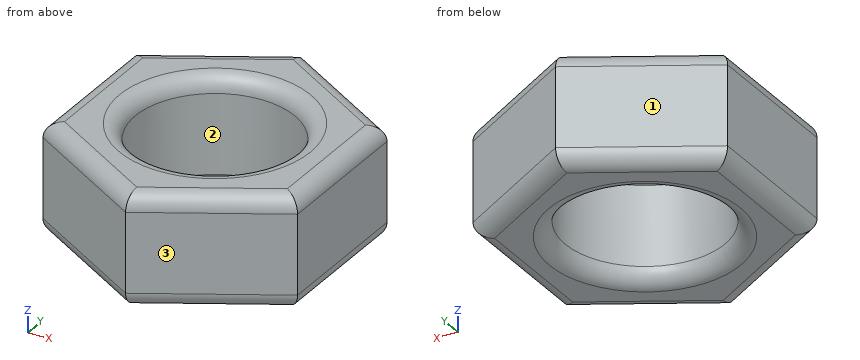
from build123d import *

# Parameters (mm, degrees)
F0_R     = 2.5
F1_DEPTH = 3.5
F2_R     = 0.5
F3_R     = 0.5


with BuildPart() as f1:
    # F0 (on Top) → F1 (new body)
    with BuildSketch(Plane.XY):
        Polygon((4, -2.309401), (4, 2.309401), (0, 4.618802), (-4, 2.309401), (-4, -2.309401), (0, -4.618802), align=None)
        Circle(F0_R, mode=Mode.SUBTRACT)
    extrude(amount=F1_DEPTH)

    # F2
    f2_edges = [f1.edges().sort_by_distance(p)[0] for p in [
        (4, 0, 3.5),
        (2, 3.464102, 3.5),
        (-2, 3.464102, 3.5),
        (-4, 0, 3.5),
        (-2, -3.464102, 3.5),
        (2, -3.464102, 3.5),
        (-2.5, 0, 3.5),
    ]]
    fillet(f2_edges, radius=F2_R)

    # F3
    f3_edges = [f1.edges().sort_by_distance(p)[0] for p in [
        (4, 0, 0),
        (2, 3.464102, 0),
        (-2, 3.464102, 0),
        (-4, 0, 0),
        (-2, -3.464102, 0),
        (2, -3.464102, 0),
        (-2.5, 0, 0),
    ]]
    fillet(f3_edges, radius=F3_R)


solid = f1.part
Design review of the part built by this model. Coordinates are the model's own, in mm. Face numbers are marked on the shaded views. Give positions to 0.01 mm unless a question says otherwise; leave off trailing zeros. Order: outer loops, then holes, each group sorted by start corner. A loop starts at its lowest first (then second) coordinate and runs counter-clockwise, first axis right, second up.
1. To check wall thickness, follow L1, parallel to Y at x = 2, z = 0.2; L2, parallel to Y at x = -1.5, z = 1.3; L3, parallel to X at y = -2, z = 1.65. State the ranges of each line that lie inside material, in increasing order.
Solution:
L1: y = -3.35 to -1.66, 1.66 to 3.35
L2: y = -3.75 to -2, 2 to 3.75
L3: x = -4 to -1.5, 1.5 to 4
2. Add section B-B, the plane z = 2.75. State the section outline as (x, y) points, then the cut area to 3 significant figures.
Solution:
outline: (-4, -2.31) - (0, -4.62) - (4, -2.31) - (4, 2.31) - (0, 4.62) - (-4, 2.31) - close; hole circle Ø5 at (0, 0)
area: 35.8 mm2
3. Add section C-C, the plane z = 3.3. State the section outline as (x, y) points.
Solution:
outline: (-3.9, -2.25) - (0, -4.5) - (3.9, -2.25) - (3.9, 2.25) - (0, 4.5) - (-3.9, 2.25) - close; hole circle Ø5.2 at (0, 0)
4. Mouldability with a two-part tool opening along Y and no side actions: class the marked faces 1, 2 and 3 as +Y half, -Y half, draft (parallel to the pull), parting line (faces both ways), or undercut.
Solution:
face 1: +Y half
face 2: undercut
face 3: -Y half
5. Add section A-A, the plane y = 0. State the section outline as (x, z) points.
Solution:
outline: (-4, 0.5) arc R0.5 ccw to (-3.5, 0) - (-3, 0) arc R0.5 ccw to (-2.5, 0.5) - (-2.5, 3) arc R0.5 ccw to (-3, 3.5) - (-3.5, 3.5) arc R0.5 ccw to (-4, 3) - close; (2.5, 0.5) arc R0.5 ccw to (3, 0) - (3.5, 0) arc R0.5 ccw to (4, 0.5) - (4, 3) arc R0.5 ccw to (3.5, 3.5) - (3, 3.5) arc R0.5 ccw to (2.5, 3) - close
6. For pin 1 Ø2 at (x, z) = (-0.5, 2) entering from +Y, flat-tipped, find the tip position at first contact; note if it passes through.
Solution:
pin 1: stops at y = 4.62
